Work out the finished part from the listing and answer in its coordinate system (mm). A direction names the side the tool comes from. Coordinates: 2 decimals unless noted, no trailing zeros. Loops run counter-clockwise (first coordinate to the right, second up) from the corner with the lowest first, then second, coordinate; pieces in that order, holes last. Notation, with made-up numbers: M 87.5,-4 L 141.5,-4 A6 ccw 141.5,0 Z; hole C 38,67.5 d11. An arc over 180 degrees is marked long. Write each question's results on one line, items separated by ' | '.
```python
from build123d import *

# Parameters (mm, degrees)
SKETCH_1_W         = 50
SKETCH_1_H         = 50
EXTRUDE_1_DEPTH    = 4
HOLE_WIZARD_M101_D = 11
FILLET_1_R         = 3
HOLE_WIZARD_M61_D  = 6.6
SKETCH_6_R         = 5
EXTRUDE_2_DEPTH    = 10


with BuildPart() as part:
    # Эскиз1 → Бобышка-Вытянуть1 (new body)
    with BuildSketch(Plane.XY):
        Rectangle(SKETCH_1_W, SKETCH_1_H)
    extrude(amount=EXTRUDE_1_DEPTH)

    # Отверстие с зазором M101 (through all)
    with Locations(Plane.XY.offset(4)):
        with Locations((0, 0)):
            Hole(HOLE_WIZARD_M101_D / 2)

    # Скругление1
    fillet_1_edges = [part.edges().sort_by_distance(p)[0] for p in [
        (25, -25, 2),
        (-25, -25, 2),
        (-25, 25, 2),
        (25, 25, 2),
    ]]
    fillet(fillet_1_edges, radius=FILLET_1_R)

    # Отверстие с зазором M61 (through all)
    with Locations(Plane(origin=(0, 0, 0), x_dir=(-1, 0, 0), z_dir=(0, 0, -1))):
        with Locations((-14.5, 14.5), (0, 0), (14.5, 14.5), (-14.5, -14.5), (14.5, -14.5)):
            Hole(HOLE_WIZARD_M61_D / 2)

    # Эскиз6 → Бобышка-Вытянуть2 (add)
    with BuildSketch(Plane.XY.offset(4)):
        Polygon((4.907477288, -8.5), (9.814954576, 0), (4.907477288, 8.5), (-4.907477288, 8.5), (-9.814954576, 0), (-4.907477288, -8.5), align=None)
        Circle(SKETCH_6_R, mode=Mode.SUBTRACT)
    extrude(amount=EXTRUDE_2_DEPTH)


solid = part.part
```
1) Find section D-D, the plane z = 10. Give the vertices of the cut face in (x, y), and give its area (3 significant figures).
Check result:
outline: M -9.81,0 L -4.91,-8.5 L 4.91,-8.5 L 9.81,0 L 4.91,8.5 L -4.91,8.5 Z; hole C 0,0 d10 | area: 172 mm^2
2) Which of the six approach directions +Z, -Z, +X, -X, +Y, -Y give full straight-line access (tool end or side, diameter ignored) to faces 1 (the face through (-7.396, -4.191, 8.93)), 2 (the face through (0, -8.5, 9)), 3 (the face through (7.396, 4.191, 8.93))?
Check result:
face 1: +Z, -X, -Y | face 2: +Z, +X, -X, -Y | face 3: +Z, +X, +Y
3) For a pull along X with two mould halves and no side action, classify faces 4 (the face through (-17.8, -14.4, 2)), 5 (the face through (7.327, -4.309, 8.93)), 6 (the face through (-11, 0, 4)) as released by +X, released by -X, zero draft, split by the parting line, or undercut.
Check result:
face 4: undercut | face 5: released by +X | face 6: zero draft
4) Find section A-A, the plane y = 14.5. Give the vertices of the cut face in (x, z), and give its area (3 significant figures).
Check result:
outline: M -25,0 L -17.8,0 L -17.8,4 L -25,4 Z; M -11.2,0 L 11.2,0 L 11.2,4 L -11.2,4 Z; M 17.8,0 L 25,0 L 25,4 L 17.8,4 Z | area: 147 mm^2
5) Find section C-C, the plane x = 0. Give the vertices of the cut face in (y, z), and give its area (3 significant figures).
Check result:
outline: M -25,0 L -5.5,0 L -5.5,4 L -5,4 L -5,14 L -8.5,14 L -8.5,4 L -25,4 Z; M 5,4 L 5.5,4 L 5.5,0 L 25,0 L 25,4 L 8.5,4 L 8.5,14 L 5,14 Z | area: 226 mm^2
6) Given pin 1 Ø10.5 at (x, y) = (14.5, -14.5) entering from +Z; pin 2 Ø2 at (x, z) = (6.5, 12.5) entering from +Y; pin 3 Ø5 at (x, z) = (-0.5, 11) entering from +Y; pin 4 Ø6 at (x, y) = (-14.5, 14.5) entering from +Z, each flat-ended and moving along its own axis, determine where each tip first touches the part or whether it passes through.
Check result:
pin 1: z = 4 | pin 2: y = 7.47 | pin 3: y = 8.5 | pin 4: through
7) Straight lines are drawn through the part: probe 1 along Y at (x, z) = (-14.5, 2.65); probe 2 along Y at (x, z) = (0, 3); probe 3 along Z at (x, y) = (-9, 15.5). For each, find the intervals that lie inside material, in ascending order. Write a range as [from, to].
Check result:
probe 1: [-25, -17.8], [-11.2, 11.2], [17.8, 25] | probe 2: [-25, -5.5], [5.5, 25] | probe 3: [0, 4]
